```python
from build123d import *

# Parameters (mm, degrees)
SKETCH_1_W          = 500
SKETCH_1_H          = 500
EXTRUDE_1_DEPTH     = 30
SKETCH_2_R          = 65
CUT_EXTRUDE_1_DEPTH = 30
FILLET_1_R          = 50
CUT_EXTRUDE_2_DEPTH = 10
SKETCH_4_R          = 20
CUT_EXTRUDE_3_DEPTH = 31


with BuildPart() as part:
    # 草图1 → 凸台-拉伸1 (new body)
    with BuildSketch(Plane(origin=(0, 0, 0), x_dir=(1, 0, 0), z_dir=(0, 1, 0))):
        Rectangle(SKETCH_1_W, SKETCH_1_H)
    extrude(amount=EXTRUDE_1_DEPTH)

    # 草图2 → 切除-拉伸1 (cut)
    with BuildSketch(Plane(origin=(0, 30, 0), x_dir=(1, 0, 0), z_dir=(0, 1, 0))):
        with Locations((150, -150)):
            Circle(SKETCH_2_R)
        with Locations((-150, -150)):
            Circle(SKETCH_2_R)
        with Locations((150, 150)):
            Circle(SKETCH_2_R)
        with Locations((-150, 150)):
            Circle(SKETCH_2_R)
    extrude(amount=-CUT_EXTRUDE_1_DEPTH, mode=Mode.SUBTRACT)

    # 圆角1
    fillet_1_edges = [part.edges().sort_by_distance(p)[0] for p in [
        (-250, 15, -250),
        (250, 15, -250),
        (250, 15, 250),
        (-250, 15, 250),
    ]]
    fillet(fillet_1_edges, radius=FILLET_1_R)

    # 草图3 → 切除-拉伸2 (cut)
    with BuildSketch(Plane(origin=(0, 30, 0), x_dir=(1, 0, 0), z_dir=(0, 1, 0))):
        Polygon((177.720371549, 0), (153.455288688, 24.265082861), (153.455288688, 12.13254143), (117.643810746, 12.13254143), (117.643810746, -12.13254143), (153.455288688, -12.13254143), (153.455288688, -24.265082861), align=None)
    extrude(amount=-CUT_EXTRUDE_2_DEPTH, mode=Mode.SUBTRACT)

    # 草图4 → 切除-拉伸3 (cut, through all)
    with BuildSketch(Plane(origin=(0, 30, 0), x_dir=(1, 0, 0), z_dir=(0, 1, 0))):
        Circle(SKETCH_4_R)
    extrude(amount=-CUT_EXTRUDE_3_DEPTH, mode=Mode.SUBTRACT)


solid = part.part
```
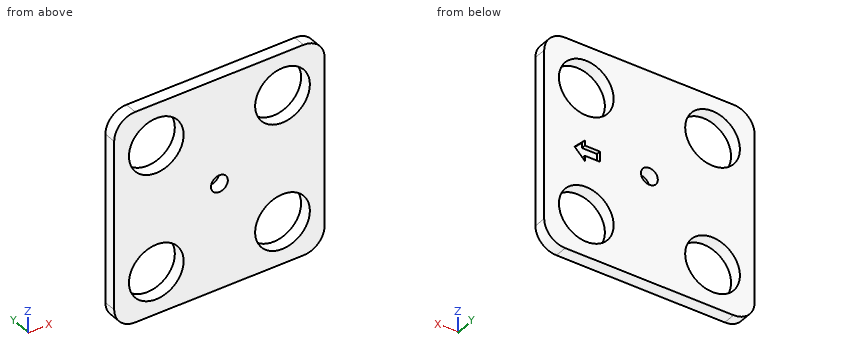
The listing builds one solid part. Answer for the finished solid, in the listing's coordinates (mm). Give positions to 0.01 mm unless a question says otherwise; leave off trailing zeros. Write each loop counter-clockwise with the first axis right and the second up, starting at its lowest first coordinate (ties: lowest second). Pieces come first, ordered by that corner, then holes. Notation, with made-up numbers: (10.5, -13.75) -> (30.5, -13.75) arc R24 ccw to (30.5, 7.25) -> close; hole circle Ø3 at (10, 69). An arc over 180 degrees is marked (long way). Use one line per item in the form item = value.
1) Section B-B on z = 150 is taken. Write down the section's boundary in (x, y).
Result:
outline = (-250, 0) -> (-215, 0) -> (-215, 30) -> (-250, 30) -> close; (-85, 0) -> (85, 0) -> (85, 30) -> (-85, 30) -> close; (215, 0) -> (250, 0) -> (250, 30) -> (215, 30) -> close
2) Section A-A on x = 0 is taken. Write down the section's boundary in (y, z), plus the area to 3 significant figures.
Result:
outline = (0, -250) -> (30, -250) -> (30, -20) -> (0, -20) -> close; (0, 20) -> (30, 20) -> (30, 250) -> (0, 250) -> close
area = 13,800 mm²
3) Section C-C on x = -150 is taken. Write down the section's boundary in (y, z), plus the area to 3 significant figures.
Result:
outline = (0, -250) -> (30, -250) -> (30, -215) -> (0, -215) -> close; (0, -85) -> (30, -85) -> (30, 85) -> (0, 85) -> close; (0, 215) -> (30, 215) -> (30, 250) -> (0, 250) -> close
area = 7,200 mm²
4) Straight lines are drawn through the part: probe 1 along Z at (x, y) = (-150, 20.25); probe 2 along X at (y, z) = (23.75, -210). For each, find the intervals that lie inside material, in ascending order.
Result:
probe_1 = -250 to -215, -85 to 85, 215 to 250
probe_2 = -248.99 to -175, -125 to 125, 175 to 248.99
5) Section D-D on y = 14 is taken. Write down the section's boundary in (x, z).
Result:
outline = (-250, -200) arc R50 ccw to (-200, -250) -> (200, -250) arc R50 ccw to (250, -200) -> (250, 200) arc R50 ccw to (200, 250) -> (-200, 250) arc R50 ccw to (-250, 200) -> close; hole circle Ø130 at (-150, -150); hole circle Ø130 at (-150, 150); hole circle Ø40 at (0, 0); hole circle Ø130 at (150, -150); hole circle Ø130 at (150, 150)
